from build123d import *

# Parameters (mm, degrees)
SKETCH1_W           = 8
SKETCH1_H           = 8
BOSS_EXTRUDE1_DEPTH = 50
SKETCH2_R           = 4
BOSS_EXTRUDE2_DEPTH = 2
CUT_EXTRUDE1_DEPTH  = 2
CHAMFER2_SIZE       = 0.15


with BuildPart() as part:
    # Sketch1 → Boss-Extrude1 (new body)
    with BuildSketch(Plane.XY):
        with Locations((4, 4)):
            Rectangle(SKETCH1_W, SKETCH1_H)
    boss_extrude1 = extrude(amount=BOSS_EXTRUDE1_DEPTH)

    # Sketch2 → Boss-Extrude2 (add)
    with BuildSketch(Plane.XY.offset(50)):
        with Locations((4, 4)):
            Circle(SKETCH2_R)
    boss_extrude2 = extrude(amount=BOSS_EXTRUDE2_DEPTH)

    # Mirror1: Boss-Extrude1, Boss-Extrude2 across Front Plane
    add(boss_extrude1.mirror(Plane.XY))
    add(boss_extrude2.mirror(Plane.XY))

    # Sketch3 → Cut-Extrude1 (cut)
    with BuildSketch(Plane.XY.offset(52)):
        Polygon((3.8, 5.7), (4.2, 5.7), (4.2, 4.2), (5.7, 4.2), (5.7, 3.8), (4.2, 3.8), (4.2, 2.3), (3.8, 2.3), (3.8, 3.8), (2.3, 3.8), (2.3, 4.2), (3.8, 4.2), align=None)
    cut_extrude1 = extrude(amount=-CUT_EXTRUDE1_DEPTH, mode=Mode.SUBTRACT)

    # Mirror3: Cut-Extrude1 across plane
    add(cut_extrude1.mirror(Plane.XY), mode=Mode.SUBTRACT)

    # Chamfer2
    chamfer2_edges = [part.edges().sort_by_distance(p)[0] for p in [
        (0, 4, 52),
        (0, 4, -52),
        (4, 5.7, 52),
        (4.2, 4.95, 52),
        (4.95, 4.2, 52),
        (5.7, 4, 52),
        (3.8, 3.05, 52),
        (3.05, 3.8, 52),
        (3.8, 4.95, 52),
        (3.05, 4.2, 52),
        (2.3, 4, 52),
        (4, 2.3, 52),
        (4.2, 3.05, 52),
        (4.95, 3.8, 52),
        (3.8, 4.95, -52),
        (3.05, 4.2, -52),
        (2.3, 4, -52),
        (4, 2.3, -52),
        (4.2, 3.05, -52),
        (4.95, 3.8, -52),
        (4, 5.7, -52),
        (4.2, 4.95, -52),
        (4.95, 4.2, -52),
        (5.7, 4, -52),
        (3.8, 3.05, -52),
        (3.05, 3.8, -52),
    ]]
    chamfer(chamfer2_edges, length=CHAMFER2_SIZE)


solid = part.part
Check sheet for the modelled part. Datum: model origin and axes. Units: mm. A direction names the side the tool comes from. Round coordinates to 2 decimals unless told otherwise and drop trailing zeros.
(1) Draft check along X on faces 4 (the flat face through (4, 8, 1)), 5 (the flat face through (4, 4, -50)), 6 (the flat face through (0, 4, 1)), 7 (the cylindrical face through (3.133, 0.095, -50.912)). Enter one of: pulls with the +X half, pulls with the -X half, needs draft (parallel to the pull), parting line crosses it, or undercut.
(2) Scan lines: probe 1 along Z at (x, y) = (0.5, 1.5); probe 2 along Z at (x, y) = (4.25, 3.75). Record each from-to range of solid material in increasing order.
(3) Access from +Z, -Z, +X, -X, +Y, -Y to the whole of each face (thin tool, end or side, straight path). Record for faces 1 (the flat face through (7, 1, -50)), 2 (the flat face through (4, 4, 50)), 3 (the flat face through (7, 1, 50)).
(4) Go/stop test with flat-tipped pins: P1, Ø1.2, axis at x = 5, z = -51.5, coming from the -Y side; P2, Ø1.2, axis at x = 3, z = -51, coming from the +Y side; P3, Ø1.6, axis at y = 3.5, z = -50.5, coming from the -X side. Record where each tip stops, or that it passes through.
Check sheet entries:
1. face 4: needs draft
1. face 5: undercut
1. face 6: pulls with the -X half
1. face 7: parting line crosses it
2. probe 1: z = -50 to 50
2. probe 2: z = -51.9 to 51.9
3. face 1: -Z, +X, -Y
3. face 2: +Z
3. face 3: +Z, +X, -Y
4. P1: stops at y = 0.02
4. P2: stops at y = 7.98
4. P3: stops at x = 0
